Model file for the job. Use its own axes, mm. Coordinates: 2 decimals unless noted, no trailing zeros. Order: outer loops, then holes, each group sorted by start corner. A loop starts at its lowest first (then second) coordinate and runs counter-clockwise, first axis right, second up. Notation, with made-up numbers: (21.25, 5.5) -> (41.25, 5.5) arc R18 ccw to (41.25, 30.5) -> close; hole circle Ø7 at (71.25, -4). An arc over 180 degrees is marked (long way). Return JSON: item names as keys, results as strings. Group by question number.
1) Pull direction Z, two halves, no side cores. Call faces 1 (the flat face through (0, -118, -3)), 2 (the flat face through (-1.5, -98.5, 197.5)), 3 (the cylindrical face through (-1.479, -110.984, 1.898)), 4 (the flat face through (-1.479, -97.067, -196.04)): +Z half, -Z half, draft (parallel to the pull), parting line (faces both ways), or undercut.
2) Cut at D-D (z = 79). Write the cut outline in (x, y), and give its area (3 significant figures).
3) Probe line 1 (Z direction, x = -0.65, y = -87); line 2 (Z direction, x = -1.7, y = -97); line 3 (Y direction, x = -1.8, z = -117). List the from-to ranges inside material, lowest first.
4) Cut at A-A (y = -84). Write the cut outline in (x, z), and give its area (3 significant figures).
5) Cut at B-B (x = -0.75). Write the cut outline in (y, z).
6) Cut at C-C (y = -60). Write the cut outline in (x, z), and give its area (3 significant figures).
7) Flat gauge pin, fed straight in: pin 1 (1 mm diameter, centred on x = -1.5, z = -16.5, fed in from +Y). Where does the tip first touch, or does it go through?
from build123d import *

# Parameters (mm, degrees)
SM_BASE_FLANGE_1_DEPTH = 3


# Sheet-metal steps are written as plain solids
with BuildPart() as part:
    # Sketch 1 → Базовая кромка1 (new body)
    with BuildSketch(Plane(origin=(0, 0, 0), x_dir=(0, 0, -1), z_dir=(1, 0, 0))):
        with BuildLine():
            Line((250, -150), (-250, -150))
            Line((-250, -150), (-143.570968245, -45.596595724))
            Line((-143.570968245, -45.596595724), (-104.305880907, -37.964235909))
            ThreePointArc((-104.305880907, -37.964235909), (0, -111), (104.305880907, -37.964235909))
            Line((104.305880907, -37.964235909), (143.570968245, -45.596595724))
            Line((143.570968245, -45.596595724), (250, -150))
        make_face()
    extrude(amount=-SM_BASE_FLANGE_1_DEPTH)


solid = part.part
Answers below:
{
 "1": {"face 1": "draft", "face 2": "+Z half", "face 3": "undercut", "face 4": "-Z half"},
 "2": {"outline": "(-3, -150) -> (0, -150) -> (0, -77.97) -> (-3, -77.97) -> close", "area": "216 mm^2"},
 "3": {"line 1": "z = -185.78 to -68.93, 68.93 to 185.78", "line 2": "z = -195.97 to -53.96, 53.96 to 195.97", "line 3": "y = -150 to -40.43"},
 "4": {"outline": "(-3, -182.72) -> (0, -182.72) -> (0, -72.56) -> (-3, -72.56) -> close; (-3, 72.56) -> (0, 72.56) -> (0, 182.72) -> (-3, 182.72) -> close", "area": "661 mm^2"},
 "5": {"outline": "(-150, -250) -> (-45.6, -143.57) -> (-37.96, -104.31) arc R111 cw to (-37.96, 104.31) -> (-45.6, 143.57) -> (-150, 250) -> close"},
 "6": {"outline": "(-3, -158.25) -> (0, -158.25) -> (0, -93.39) -> (-3, -93.39) -> close; (-3, 93.39) -> (0, 93.39) -> (0, 158.25) -> (-3, 158.25) -> close", "area": "389 mm^2"},
 "7": {"pin 1": "stops at y = -109.69"}
}
